The model under review builds one solid part; all positions refer to its coordinate system, in mm. A direction names the side the tool comes from. Coordinates: 2 decimals unless noted, no trailing zeros. Order: outer loops, then holes, each group sorted by start corner. A loop starts at its lowest first (then second) coordinate and runs counter-clockwise, first axis right, second up.
Autodesk Inventor part; units mm, degrees
ref_plane "YZ Plane" through (0, 0, 0) normal (1, 0, 0) x (0, 1, 0)
ref_plane "XZ Plane" through (0, 0, 0) normal (0, 1, 0) x (-1, 0, 0)
ref_plane "XY Plane" through (0, 0, 0) normal (0, 0, 1) x (1, 0, 0)
sketch "Sketch1" plane through (0, 0, 0) normal (0, 0, 1) x (1, 0, 0)
  arc A0 (-32.5521, -67.5675) -> (32.5521, 67.5675) centre (0, 0) ccw
  circle A1 centre (0, 0) radius 25
  arc A2 (-473.7534, 311.4911) -> (-538.8576, 176.3561) centre (-506.3055, 243.9236) ccw
  circle A3 centre (-506.3055, 243.9236) radius 25
  line L0 (-473.7534, 311.4911) -> (32.5521, 67.5675)
  line L1 (-538.8576, 176.3561) -> (-32.5521, -67.5675)
  dimension "d0" = 150
  dimension "d1" = 50
  dimension "d2" = 150
  dimension "d3" = 50
  dimension "d4" = 562
extrude "Extrusion1" add sketch "Sketch1" along normal blind 207
sketch "Sketch2" plane through (-473.7534, 311.4911, 207) normal (0.4340278, 0.9008995, 0) x (0.9008995, -0.4340278, 0)
  line L0 (116.8603, 30) -> (-116.8603, 30)
  line L1 (-116.8603, 30) -> (-116.8603, 177)
  line L2 (-116.8603, 177) -> (116.8603, 177)
  line L3 (116.8603, 177) -> (116.8603, 30)
  line L4 (0, 207) -> (0, 0)
  line L5 (116.8603, 30) -> (-116.8603, 177) construction
  line L6 (-116.8603, 30) -> (116.8603, 177) construction
  line L7 (-75, 0) -> (0, 0)
  point P0 (562, 207)
  point P1 (0, 103.5)
  dimension "d7" = 30
extrude "Extrusion2" cut sketch "Sketch2" against normal blind 207
sketch "Sketch3" plane through (32.5521, 67.5675, 207) normal (0.4340278, 0.9008995, 0) x (0.9008995, -0.4340278, 0)
  line L0 (110.57, 177) -> (-160.57, 177)
  line L1 (-160.57, 177) -> (-160.57, 30)
  line L2 (-160.57, 30) -> (110.57, 30)
  line L3 (110.57, 30) -> (110.57, 177)
  line L4 (-25, 0) -> (-25, 207)
  line L5 (110.57, 177) -> (-160.57, 30) construction
  line L6 (-160.57, 177) -> (110.57, 30) construction
  point P0 (0, 207)
  point P1 (-25, 103.5)
  dimension "d10" = 30
extrude "Extrusion3" cut sketch "Sketch3" against normal blind 207
properties part number "SECOND ARM"
(1) Consider section B-B (x = -500). Give the boundary of the cut face in (y, z), then the cut area to 3 significant figures.
(2) Insertion check: pin 1 Ø1 at (y, z) = (161, 32.5) entering from -X; pin 2 Ø6 at (x, z) = (-201, 70) entering from -Y; pin 3 Ø4 at (x, z) = (-309.5, 22.5) entering from -Y. Each pin has a flat end and moves straight along its axis. Give the tip position at first contact, or say it passes through.
(3) Consider section C-C (y = -46). Give the boundary of the cut face in (x, z).
(4) The part is to be moulded in two halves that separate along Z. For faces 1 (the face through (-37, 19, 30)), 2 (the face through (-258, 125, 207)), 3 (the face through (-224.145, 191.237, 102.051)), 4 (the face through (-467, 226, 177)), say which applies: +Z half, -Z half, draft (parallel to the pull), parting line (faces both ways), or undercut.
(5) Wall thickness on line 1 (Z direction, x = 46, y = 37.5); line 2 (X direction, y = 0, z = 200); line 3 (Y direction, x = 0, z = 22): over which ranges is each line inside the solid? List them lowest first.
(6) Consider section A-A (y = 10). Give the boundary of the cut face in (x, z), then the cut area to 3 significant figures.
(7) Consider section D-D (z = 19.5). Give the boundary of the cut face in (x, y), then the cut area to 3 significant figures.
(8) Tool access review of faces 5 (the face through (-258, 125, 0)), 6 (the face through (-469, 227, 30)), 7 (the face through (-144.2, 70.64, 102.47)): name each direction out of +Z, -Z, +X, -X, +Y, -Y from which nothing blocks a thin tool from reaching the whole face with its end or side.
Findings:
1. outline: (157.64, 0) - (219.73, 0) - (219.73, 30) - (157.64, 30) - close; (157.64, 177) - (219.73, 177) - (219.73, 207) - (157.64, 207) - close; (268.12, 0) - (318.66, 0) - (318.66, 30) - (268.12, 30) - close; (268.12, 177) - (318.66, 177) - (318.66, 207) - (268.12, 207) - close
1. area: 6,760 mm2
2. pin 1: stops at x = -416.78
2. pin 2: stops at y = 12.14
2. pin 3: stops at y = 64.89
3. outline: (-77.32, 0) - (59.24, 0) - (59.24, 30) - (-77.32, 30) - close; (-77.32, 177) - (59.24, 177) - (59.24, 207) - (-77.32, 207) - close
4. face 1: undercut
4. face 2: +Z half
4. face 3: draft
4. face 4: undercut
5. line 1: z = 0 to 30, 177 to 207
5. line 2: x = -172.8 to -25, 25 to 75
5. line 3: y = -75 to -25, 25 to 83.25
6. outline: (-193.56, 0) - (-22.91, 0) - (-22.91, 30) - (-173.42, 30) - (-173.42, 177) - (-22.91, 177) - (-22.91, 207) - (-193.56, 207) - close; (22.91, 0) - (74.33, 0) - (74.33, 30) - (22.91, 30) - close; (22.91, 177) - (74.33, 177) - (74.33, 207) - (22.91, 207) - close
6. area: 16,300 mm2
7. outline: (-538.86, 176.36) - (-32.55, -67.57) arc R75 ccw to (32.55, 67.57) - (-473.75, 311.49) arc R75 ccw to start; hole circle Ø50 at (-506.31, 243.92); hole circle Ø50 at (0, 0)
7. area: 98,000 mm2
8. face 5: -Z, +X, -X, +Y, -Y
8. face 6: -X, +Y
8. face 7: +X, -Y
